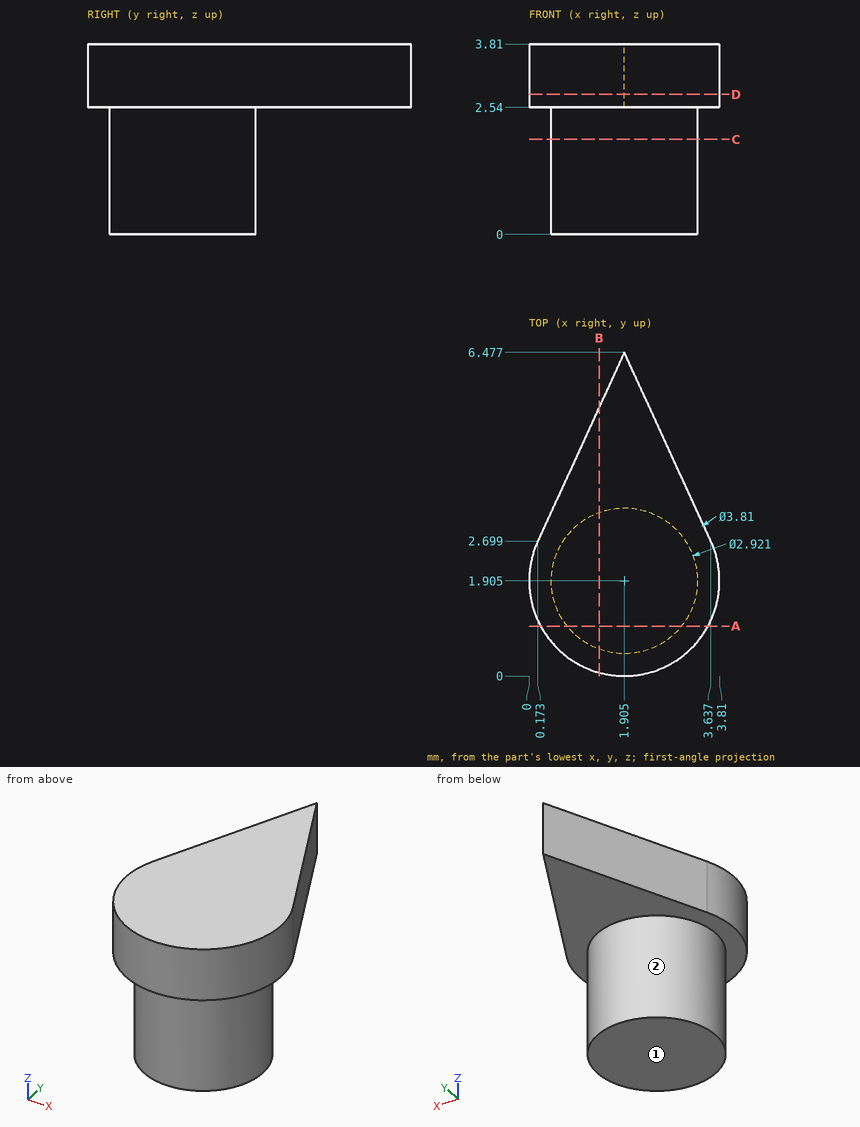
Input: dimensioned drawing with shaded views. Units: mm. Origin: part minimum x, y, z. A direction names the side the tool comes from. Round coordinates to 2 decimals unless told otherwise and drop trailing zeros. Order: outer loops, then holes, each group sorted by start corner. A loop starts at its lowest first (then second) coordinate and runs counter-clockwise, first axis right, second up. Notation, with made-up numbers: (55.5, 79.25) -> (65.5, 79.25) arc R22 ccw to (65.5, 106.25) -> close; hole circle Ø7 at (31.5, 33.25). An arc over 180 degrees is marked (long way). One line per item, written item: value. Start each with the question number.
Q1. Material intervals for probe 1 along Z at (x, y) = (0.7, 0.5); probe 2 along X at (y, z) = (2, 2.75); probe 3 along Y at (x, z) = (2.75, 1.9) (1 decimal), sorted ascending.
Q2. Section query C-C (z = 1.9). Return the cut outline in (x, y) (1 decimal).
Q3. Pin query (flat end, axial travel): pin 1 (1.5 mm diameter, centred on y = 1, z = 3, fed in from -X); pin 2 (2 mm diameter, centred on y = 3.5, z = 0.5, fed in from -X). Return the tip coordinate at first contact, or that it passes through.
Q4. Section query A-A (y = 1). Return the cut outline in (x, z), plus the area to 3 significant figures.
Q5. Section query D-D (z = 2.8). Return the cut outline in (x, y) (1 decimal).
Q6. Access query for the marked faces 1 and 2. Directions: +Z, -Z, +X, -X, +Y, -Y. A direction counts if a zero-diameter tool reaches every point of the face in a straight line with its end or side. Return the directions, or none.
Q7. Section query B-B (x = 1.4). Return the cut outline in (y, z) (1 decimal), plus the area to 3 significant figures.
Findings below:
1. probe 1: 2.54 to 3.81
1. probe 2: 0 to 3.81
1. probe 3: 0.7 to 3.1
2. outline: circle Ø2.9 at (1.9, 1.9)
3. pin 1: x = 0.01
3. pin 2: x = 0.57
4. outline: (0.23, 2.54) -> (0.76, 2.54) -> (0.76, 0) -> (3.05, 0) -> (3.05, 2.54) -> (3.58, 2.54) -> (3.58, 3.81) -> (0.23, 3.81) -> close
4. area: 10.1 mm²
5. outline: (0.2, 2.7) arc R1.9 ccw (long way) to (3.6, 2.7) -> (1.9, 6.5) -> close
6. face 1: -Z, +X, -X, +Y, -Y
6. face 2: -Z
7. outline: (0.1, 2.5) -> (0.5, 2.5) -> (0.5, 0) -> (3.3, 0) -> (3.3, 2.5) -> (5.4, 2.5) -> (5.4, 3.8) -> (0.1, 3.8) -> close
7. area: 13.7 mm²
